Geometry: final body of the model. Coordinates: model frame, mm. A direction names the side the tool comes from. Give positions to 0.01 mm unless a question says otherwise; leave off trailing zeros. Write each loop counter-clockwise with the first axis right and the second up, starting at its lowest first coordinate (ties: lowest second). Pieces come first, ordered by that corner, then holes. Notation, with made-up numbers: (23, 32) -> (45, 32) arc R5 cw to (45, 37) -> close; hole circle Ø2 at (24.25, -10). An arc over 180 degrees is marked (long way). Answer as a JSON object with one key per item and string values. Group by question number.
(1) Section query A-A on z = -67. Output: boundary loops of the cut face in (x, y) (3 decimals).
(2) Material intervals for probe 1 along X at (y, z) = (-2, -475); probe 2 along Z at (x, y) = (0, -10.6), sorted ascending.
(3) Set-up query: faces 1 (the face through (0, 12.7, -376)), 2 (the face through (0, -9.652, -376)). Return all of +Z, -Z, +X, -X, +Y, -Y with unobstructed straight access to the full face (end or side cutting, diameter ignored); none if empty.
(4) Draft query along X for faces 3 (the face through (11, 0, -762)), 4 (the face through (-12.7, 0, -376)), 5 (the face through (0, 9.652, -376)). Return one class per face: +X half, -X half, draft (parallel to the pull), parting line (faces both ways), or undercut.
(5) Section query B-B on y = -2. Output: boundary loops of the cut face in (x, z).
(6) Section query C-C on x = 0. Output: boundary loops of the cut face in (y, z), plus the area to 3 significant figures.
from build123d import *

# Parameters (mm, degrees)
F0_W     = 25.4
F0_H     = 25.4
F1_DEPTH = 762
F2_R     = 3.175
F3_T     = -3.048
F4_R     = 4.5
F5_DEPTH = 12.7


with BuildPart() as f1:
    # F0 (on Top) → F1 (new body)
    with BuildSketch(Plane.XY):
        Rectangle(F0_W, F0_H)
    extrude(amount=-F1_DEPTH)

    # F2
    f2_edges = [f1.edges().sort_by_distance(p)[0] for p in [
        (-12.7, 12.7, -381),
        (-12.7, -12.7, -381),
        (12.7, 12.7, -381),
        (12.7, -12.7, -381),
    ]]
    fillet(f2_edges, radius=F2_R)

    # F3
    f3_openings = [f1.faces().sort_by_distance(p)[0] for p in [
        (0, 0, 0),
        (0, 0, -762),
    ]]
    offset(amount=F3_T, openings=f3_openings)

    # F4 (on Front) → F5 (cut, through all)
    with BuildSketch(Plane.XZ):
        with Locations((0, -660.4)):
            Circle(F4_R)
    extrude(amount=F5_DEPTH, mode=Mode.SUBTRACT)


solid = f1.part
Answer list:
{
 "1": {"outline": "(-12.7, -9.525) arc R3.175 ccw to (-9.525, -12.7) -> (9.525, -12.7) arc R3.175 ccw to (12.7, -9.525) -> (12.7, 9.525) arc R3.175 ccw to (9.525, 12.7) -> (-9.525, 12.7) arc R3.175 ccw to (-12.7, 9.525) -> close; hole (-9.652, -9.525) arc R0.127 ccw to (-9.525, -9.652) -> (9.525, -9.652) arc R0.127 ccw to (9.652, -9.525) -> (9.652, 9.525) arc R0.127 ccw to (9.525, 9.652) -> (-9.525, 9.652) arc R0.127 ccw to (-9.652, 9.525) -> close"},
 "2": {"probe 1": "-12.7 to -9.65, 9.65 to 12.7", "probe 2": "-762 to -664.9, -655.9 to 0"},
 "3": {"face 1": "+Z, -Z, +X, -X, +Y", "face 2": "+Z, -Z"},
 "4": {"face 3": "draft", "face 4": "-X half", "face 5": "undercut"},
 "5": {"outline": "(-12.7, -762) -> (-9.65, -762) -> (-9.65, 0) -> (-12.7, 0) -> close; (9.65, -762) -> (12.7, -762) -> (12.7, 0) -> (9.65, 0) -> close"},
 "6": {"outline": "(-12.7, -762) -> (-9.65, -762) -> (-9.65, -664.9) -> (-12.7, -664.9) -> close; (-12.7, -655.9) -> (-9.65, -655.9) -> (-9.65, 0) -> (-12.7, 0) -> close; (9.65, -762) -> (12.7, -762) -> (12.7, 0) -> (9.65, 0) -> close", "area": "4,620 mm2"}
}
